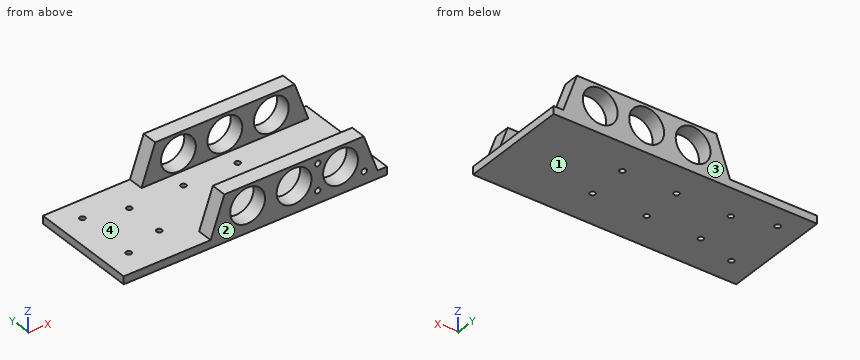
```python
from build123d import *

# Parameters (mm, degrees)
SKETCH_1_R          = 11.25
EXTRUDE_1_DEPTH     = 35
SKETCH_2_W          = 25
SKETCH_2_H          = 50
CUT_EXTRUDE1_DEPTH  = 147.905581923
SKETCH1_W           = 30
SKETCH1_H           = 70
BOSS_EXTRUDE1_DEPTH = 5
SKETCH3_R           = 1.75
CUT_EXTRUDE4_DEPTH  = 10
SKETCH_3_R          = 1.75
CUT_EXTRUDE_2_DEPTH = 10


with BuildPart() as part:
    # Эскиз1 → Бобышка-Вытянуть1 (new, symmetric)
    with BuildSketch(Plane(origin=(0, 0, 0), x_dir=(1, 0, 0), z_dir=(0, 1, 0))):
        Polygon((-60, -2.5), (-53.870442851, -2.5), (-45, -27.5), (45, -27.5), (53.870442851, -2.5), (60, -2.5), (60, 2.5), (-60, 2.5), (-80, 2.5), (-80, -2.5), align=None)
        with Locations(Location((0, -14.5, 0), (0, 0, 270))):
            Circle(SKETCH_1_R, mode=Mode.SUBTRACT)
        with Locations(Location((30, -14.5, 0), (0, 0, 270))):
            Circle(SKETCH_1_R, mode=Mode.SUBTRACT)
        with Locations(Location((-30, -14.5, 0), (0, 0, 90))):
            Circle(SKETCH_1_R, mode=Mode.SUBTRACT)
    extrude(amount=EXTRUDE_1_DEPTH, both=True)

    # Эскиз2 → Cut-Extrude1 (cut, through all)
    with BuildSketch(Plane.ZY.offset(80)):
        with Locations((15, 0)):
            Rectangle(SKETCH_2_W, SKETCH_2_H)
    extrude(amount=-CUT_EXTRUDE1_DEPTH, mode=Mode.SUBTRACT)

    # Sketch1 → Boss-Extrude1 (add)
    with BuildSketch(Plane(origin=(0, 0, -2.5), x_dir=(-1, 0, 0), z_dir=(0, 0, -1))):
        with Locations((95, 0)):
            Rectangle(SKETCH1_W, SKETCH1_H)
    extrude(amount=-BOSS_EXTRUDE1_DEPTH)

    # Sketch3 → Cut-Extrude4 (cut)
    with BuildSketch(Plane.XZ.offset(35)):
        with Locations(Location((45.3, 5.5, 0), (0, 0, 270))):
            Circle(SKETCH3_R)
        with Locations(Location((15.3, 22.5, 0), (0, 0, 270))):
            Circle(SKETCH3_R)
        with Locations(Location((15.3, 5.5, 0), (0, 0, 270))):
            Circle(SKETCH3_R)
    extrude(amount=-CUT_EXTRUDE4_DEPTH, mode=Mode.SUBTRACT)

    # Эскиз3 → Вырез-Вытянуть2 (cut)
    with BuildSketch(Plane(origin=(0, 0, -2.5), x_dir=(-1, 0, 0), z_dir=(0, 0, -1))):
        with Locations((0, -12)):
            Circle(SKETCH_3_R)
        with Locations((35, -12)):
            Circle(SKETCH_3_R)
        with Locations((70, -12)):
            Circle(SKETCH_3_R)
        with Locations((35, 13.91)):
            Circle(SKETCH_3_R)
        with Locations((70, 13.91)):
            Circle(SKETCH_3_R)
        with Locations((0, 13.91)):
            Circle(SKETCH_3_R)
        with Locations((95, 20.955)):
            Circle(SKETCH_3_R)
        with Locations((95, -19.045)):
            Circle(SKETCH_3_R)
    extrude(amount=-CUT_EXTRUDE_2_DEPTH, mode=Mode.SUBTRACT)


solid = part.part
```
For this review, take the finished solid that the model builds, in its own axes (mm). Face numbers are marked on the shaded views. Give positions to 0.01 mm unless a question says otherwise; leave off trailing zeros. Loops run counter-clockwise (first coordinate to the right, second up) from the corner with the lowest first, then second, coordinate; pieces in that order, holes last. Notation, with made-up numbers: M 41.5,47.25 L 83.5,47.25 A16 cw 83.5,65.25 Z; hole C 67,61 d1. An arc over 180 degrees is marked long. One line per item, written item: value. Start each with the question number.
Q1. Add section D-D (y = -2). Give the boundary of the cut face in (x, z).
Q2. Add section B-B (x = -70). Give the boundary of the cut face in (y, z).
Q3. Draft analysis for pull direction Y (two halves, no side actions). For the marked faces 1, 2, 3 and 4, state which applies: released by +Y, released by -Y, zero draft, split by the parting line, or undercut.
Q4. Add section C-C (z = 16.5). Count the separate pieces of the cut face and the enclosed holes in it, and give its area (3 significant figures).
Q5. Add section A-A (x = 0). Give the boundary of the cut face in (y, z), and give its area (3 significant figures).
Q6. For L1, parallel to Y at x = -35, z = -0.9; L2, parallel to Z at x = 0, y = 27.75; L3, parallel to X at y = 28.5, z = 24.25, list the stretches that pass through material, from the lowest coordinate up.
Q7. Clearance check with flat-ended pins moving along their axes: pin 1 Ø5 at (x, y) = (37, 11.5) entering from +Z; pin 2 Ø3 at (x, z) = (45.3, 5.5) entering from -Y. State where each tip first meets the part, or that it passes through.
Reply:
1. outline: M -110,-2.5 L 60,-2.5 L 60,2.5 L -110,2.5 Z
2. outline: M -35,-2.5 L -13.75,-2.5 L -13.75,2.5 L -35,2.5 Z; M -10.25,-2.5 L 12.16,-2.5 L 12.16,2.5 L -10.25,2.5 Z; M 15.66,-2.5 L 35,-2.5 L 35,2.5 L 15.66,2.5 Z
3. face 1: zero draft
3. face 2: released by -Y
3. face 3: released by +Y
3. face 4: undercut
4. separate pieces: 8
4. enclosed holes: 0
4. area: 628 mm²
5. outline: M -35,-2.5 L -13.75,-2.5 L -13.75,2.5 L -25,2.5 L -25,3.25 L -35,3.25 Z; M -35,25.75 L -25,25.75 L -25,27.5 L -35,27.5 Z; M -10.25,-2.5 L 12.16,-2.5 L 12.16,2.5 L -10.25,2.5 Z; M 15.66,-2.5 L 35,-2.5 L 35,3.25 L 25,3.25 L 25,2.5 L 15.66,2.5 Z; M 25,25.75 L 35,25.75 L 35,27.5 L 25,27.5 Z
5. area: 365 mm²
6. L1: -35 to -13.75, -10.25 to 12.16, 15.66 to 35
6. L2: -2.5 to 3.25, 25.75 to 27.5
6. L3: -46.15 to -35.61, -24.39 to -5.61, 5.61 to 24.39, 35.61 to 46.15
7. pin 1: z = 2.5
7. pin 2: y = 25
